```python
from build123d import *

# Parameters (mm, degrees)
SKETCH1_W           = 30
SKETCH1_H           = 1.5
SKETCH1_W_2         = 7
SKETCH1_H_2         = 11
SKETCH1_W_3         = 4
SKETCH1_H_3         = 8
BOSS_EXTRUDE1_DEPTH = 4
SKETCH2_W           = 2
SKETCH2_H           = 1.5
BOSS_EXTRUDE2_DEPTH = 2
SKETCH3_W           = 2
SKETCH3_H           = 1.5
BOSS_EXTRUDE3_DEPTH = 2


with BuildPart() as part:
    # Sketch1 → Boss-Extrude1 (new body)
    # profile 1 of 2: a face of its own
    with BuildSketch(Plane(origin=(0, 0, 0), x_dir=(1, 0, 0), z_dir=(0, 1, 0))):
        with Locations((18.5, 0)):
            Rectangle(SKETCH1_W, SKETCH1_H)
    # profile 2 of 2: a face of its own
    with BuildSketch(Plane(origin=(0, 0, 0), x_dir=(1, 0, 0), z_dir=(0, 1, 0))):
        Rectangle(SKETCH1_W_2, SKETCH1_H_2)
        Rectangle(SKETCH1_W_3, SKETCH1_H_3, mode=Mode.SUBTRACT)
    extrude(amount=BOSS_EXTRUDE1_DEPTH)

    # Sketch2 → Boss-Extrude2 (add)
    with BuildSketch(Plane.XZ):
        with Locations((15, 0)):
            Rectangle(SKETCH2_W, SKETCH2_H)
    extrude(amount=BOSS_EXTRUDE2_DEPTH)

    # Sketch3 → Boss-Extrude3 (add)
    with BuildSketch(Plane(origin=(0, 0, 0), x_dir=(-1, 0, 0), z_dir=(0, -1, 0))):
        with Locations((-4.5, 0)):
            Rectangle(SKETCH3_W, SKETCH3_H)
    extrude(amount=BOSS_EXTRUDE3_DEPTH)


solid = part.part
```
Source: CAD feature listing. Evaluate the final solid. Frame: model axes, mm. A direction names the side the tool comes from. Round coordinates to 2 decimals unless told otherwise and drop trailing zeros. Loops run counter-clockwise (first coordinate to the right, second up) from the corner with the lowest first, then second, coordinate; pieces in that order, holes last. Notation, with made-up numbers: M 88.25,-13.5 L 135.25,-13.5 A25 ccw 135.25,8.5 Z; hole C -5.5,17 d4. An arc over 180 degrees is marked long. Use a Markdown table: item, result. Add a question column.
1. Section query A-A on z = 2.5. Return the cut outline in (x, y).
2. Contact query for flat-ended pins moving along their axis: P1, Ø2, axis at y = 2.5, z = 3.5, coming from the +X side; P2, Ø0.8, axis at y = -1, z = 0.5, coming from the -X side; P3, Ø0.8, axis at x = 25.5, z = 0.5, coming from the -Y side. Output: stop coordinate, or through.
3. Section query B-B on y = -1. Return the cut outline in (x, z), then the cut area to 3 significant figures.
4. Line query: line 1 (X direction, y = 3.05, z = -3); line 2 (X direction, y = 3.2, z = -0.25); line 3 (Z direction, x = -1, y = 1.3). Output: solid intervals per line, ascending.
5. Mould query, pull axis Z, two halves, no side actions, for faces 1 (the flat face through (14, -1, 0)), 2 (the flat face through (19, 2, -0.75)), 3 (the flat face through (-2, 2, 0)). Classes: pulls with the +Z half, pulls with the -Z half, needs draft (parallel to the pull), parting line crosses it, or undercut.
6. Section query D-D on x = 15. Return the cut outline in (y, z).
7. Section query C-C on y = 2.3. Return the cut outline in (x, z), then the cut area to 3 significant figures.
8. Reachability of faces 4 (the flat face through (3.5, -1, 0)), 5 (the flat face through (3.5, 2, -3)), 6 (the flat face through (2, 2, 0)), 7 (the flat face through (10, 0, 0)) from +Z, -Z, +X, -X, +Y, -Y: full face, straight path, thin tool, end or side. Return the list, or none.
Reported:
| question | item | result |
|---|---|---|
| 1 | outline | M -3.5,0 L -2,0 L -2,4 L -3.5,4 Z; M 2,0 L 3.5,0 L 3.5,4 L 2,4 Z |
| 2 | P1 | stops at x = 3.5 |
| 2 | P2 | stops at x = 3.5 |
| 2 | P3 | stops at y = 0 |
| 3 | outline | M 3.5,-0.75 L 5.5,-0.75 L 5.5,0.75 L 3.5,0.75 Z; M 14,-0.75 L 16,-0.75 L 16,0.75 L 14,0.75 Z |
| 3 | area | 6.00 mm² |
| 4 | line 1 | x = -3.5 to -2, 2 to 3.5 |
| 4 | line 2 | x = -3.5 to -2, 2 to 33.5 |
| 4 | line 3 | z = -5.5 to -4, 4 to 5.5 |
| 5 | face 1 | needs draft |
| 5 | face 2 | pulls with the -Z half |
| 5 | face 3 | undercut |
| 6 | outline | M -2,-0.75 L 4,-0.75 L 4,0.75 L -2,0.75 Z |
| 7 | outline | M -3.5,-5.5 L 3.5,-5.5 L 3.5,-0.75 L 33.5,-0.75 L 33.5,0.75 L 3.5,0.75 L 3.5,5.5 L -3.5,5.5 Z; hole M -2,-4 L 2,-4 L 2,4 L -2,4 Z |
| 7 | area | 90.0 mm² |
| 8 | face 4 | +Z, -Z, -X, -Y |
| 8 | face 5 | -Z, +X, +Y, -Y |
| 8 | face 6 | +Y, -Y |
| 8 | face 7 | +Z, -Z, -Y |
